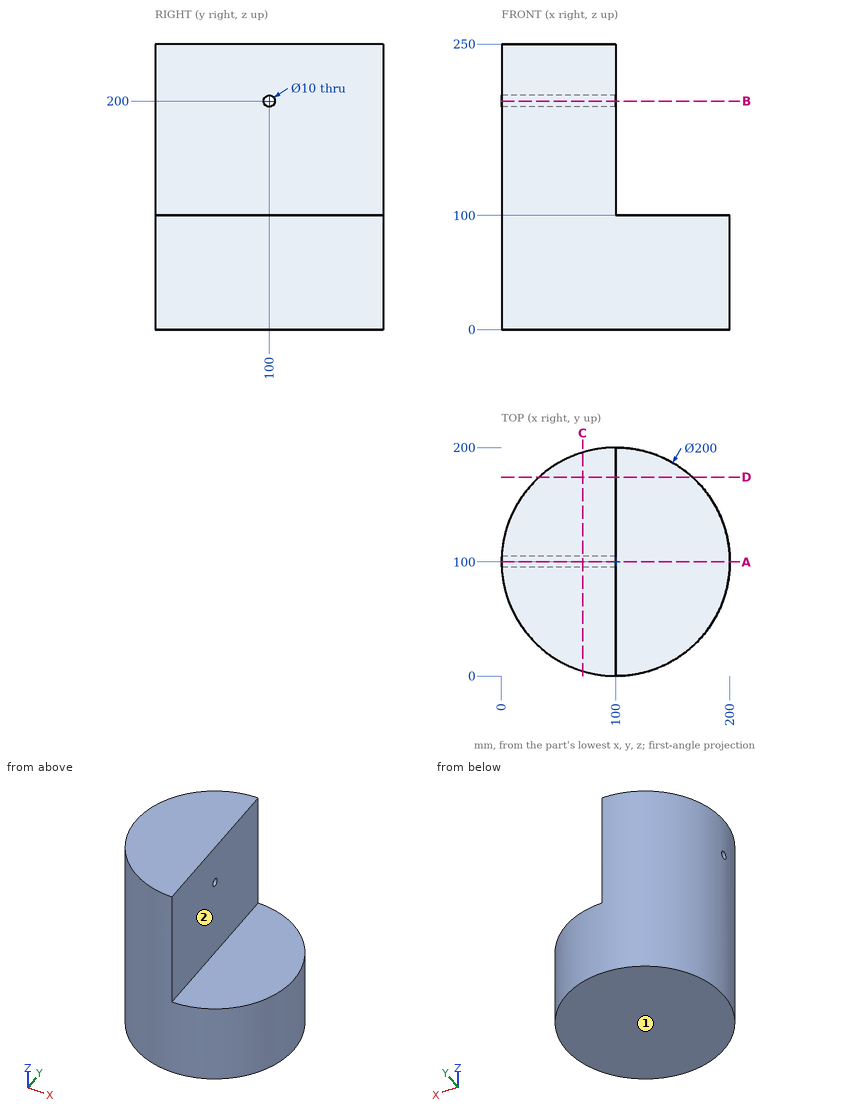
Can you work these out from the drawing? Everything is in mm from the part's minimum corner. A direction names the side the tool comes from. Coordinates: 2 decimals unless noted, no trailing zeros. Order: outer loops, then holes, each group sorted by start corner. A loop starts at its lowest first (then second) coordinate and runs counter-clockwise, first axis right, second up. Notation, with made-up numbers: (-40, -18) -> (-3, -18) arc R24 ccw to (-3, 5) -> close; hole circle Ø11 at (-34.75, 0.5). An arc over 180 degrees is marked (long way). Use one line per item in the form item = value.
Q1. Imagine slicing it at A-A, the plane y = 100. List the corners of the cut face in (x, z) for me.
From the geometry:
outline = (0, 0) -> (200, 0) -> (200, 100) -> (100, 100) -> (100, 195) -> (0, 195) -> close; (0, 205) -> (100, 205) -> (100, 250) -> (0, 250) -> close
Q2. Imagine slicing it at D-D, the plane y = 174. List the corners of the cut face in (x, z) for me.
From the geometry:
outline = (32.74, 0) -> (167.26, 0) -> (167.26, 100) -> (100, 100) -> (100, 250) -> (32.74, 250) -> close
Q3. I need wall thicknesses on L1, parallel to Z at x = 115.5, y = 12.5; L2, parallel to Y at x = 38.5, z = 200; L3, parallel to Y at x = 48, z = 200. Which ranges of each line are inside material? Lowest first, please.
From the geometry:
L1 = 0 to 100
L2 = 21.15 to 95, 105 to 178.85
L3 = 14.58 to 95, 105 to 185.42
Q4. Imagine slicing it at B-B, the plane z = 200. List the corners of the cut face in (x, y) for me, then the cut area to 3 significant figures.
From the geometry:
outline = (0.13, 95) arc R100 ccw to (100, 0) -> (100, 95) -> close; (0.13, 105) -> (100, 105) -> (100, 200) arc R100 ccw to start
area = 14,700 mm²
Q5. Imagine slicing it at C-C, the plane x = 71. List the corners of the cut face in (y, z) for me.
From the geometry:
outline = (4.3, 0) -> (195.7, 0) -> (195.7, 250) -> (4.3, 250) -> close; hole circle Ø10 at (100, 200)
Q6. Which directions (+Z, -Z, +X, -X, +Y, -Y) give clear straight access to the entire face, cutting with the end or side of a thin tool? Please do the marked faces 1 and 2.
From the geometry:
face_1 = -Z, +X, -X, +Y, -Y
face_2 = +Z, +X, +Y, -Y
Q7. Will these pins go through, and if not, where does the flat tip stop? P1, Ø2, axis at x = 26, z = 160.5, coming from the -Y side; P2, Ø12, axis at y = 152.5, z = 112, coming from the -X side; P3, Ø6, axis at y = 73.5, z = 169.5, coming from the +X side; P4, Ø6, axis at y = 100, z = 200, coming from the -X side (3 decimals).
From the geometry:
P1 = 31.66
P2 = 11.47
P3 = 100
P4 = through
